Model file for the job. Use its own axes, mm. Give positions to 0.01 mm unless a question says otherwise; leave off trailing zeros. Answer as CSV lines item,"result". Start each with the question number.
Item 1: Pin check, flat tips, straight feed: pin 1 (0.8 mm diameter, centred on y = -234.5, z = 4, fed in from +X); pin 2 (0.8 mm diameter, centred on x = 4, y = -162, fed in from -Z); pin 3 (1.3 mm diameter, centred on x = -1.5, y = -277.5, fed in from +Z). Stop position of each tip, or through.
Item 2: Saw through at A-A on y = -317. State how many separate pieces and enclosed holes the cut face has, plus the area to 3 significant figures.
Item 3: Drill centre lines: L1, parallel to Z at x = 0, y = -327.5; L2, parallel to X at y = -107.5, z = 4.25; L3, parallel to Z at x = 3.25, y = -151. Where is each one in solid material? Low to high. Write a range as from..to.
from build123d import *

# Parameters (mm, degrees)
F0_R     = 2.1
F1_DEPTH = 460


with BuildPart() as f1:
    # F0 (on Front) → F1 (new body)
    with BuildSketch(Plane.XZ):
        with BuildLine():
            Line((-4.64, 10), (-9, 10))
            ThreePointArc((-9, 10), (-9.707107, 9.707107), (-10, 9))
            Line((-10, 9), (-10, 4.64))
            Line((-10, 4.64), (-8.2, 2.84))
            Line((-8.2, 2.84), (-8.2, 5.49934))
            Line((-8.2, 5.49934), (-6.56, 5.49934))
            Line((-6.56, 5.49934), (-3.90066, 2.84))
            Line((-3.90066, 2.84), (-3.90066, 0.15))
            Line((-3.90066, 0.15), (-3.75066, 0))
            Line((-3.75066, 0), (-3.90066, -0.15))
            Line((-3.90066, -0.15), (-3.90066, -2.84))
            Line((-3.90066, -2.84), (-6.56, -5.49934))
            Line((-6.56, -5.49934), (-8.2, -5.49934))
            Line((-8.2, -5.49934), (-8.2, -2.84))
            Line((-8.2, -2.84), (-10, -4.64))
            Line((-10, -4.64), (-10, -9))
            ThreePointArc((-10, -9), (-9.707107, -9.707107), (-9, -10))
            Line((-9, -10), (-4.64, -10))
            Line((-4.64, -10), (-2.84, -8.2))
            Line((-2.84, -8.2), (-5.49934, -8.2))
            Line((-5.49934, -8.2), (-5.49934, -6.56))
            Line((-5.49934, -6.56), (-2.84, -3.90066))
            Line((-2.84, -3.90066), (-0.15, -3.90066))
            Line((-0.15, -3.90066), (0, -3.75066))
            Line((0, -3.75066), (0.15, -3.90066))
            Line((0.15, -3.90066), (2.84, -3.90066))
            Line((2.84, -3.90066), (5.49934, -6.56))
            Line((5.49934, -6.56), (5.49934, -8.2))
            Line((5.49934, -8.2), (2.84, -8.2))
            Line((2.84, -8.2), (4.64, -10))
            Line((4.64, -10), (9, -10))
            ThreePointArc((9, -10), (9.707107, -9.707107), (10, -9))
            Line((10, -9), (10, -4.64))
            Line((10, -4.64), (8.2, -2.84))
            Line((8.2, -2.84), (8.2, -5.49934))
            Line((8.2, -5.49934), (6.56, -5.49934))
            Line((6.56, -5.49934), (3.90066, -2.84))
            Line((3.90066, -2.84), (3.90066, -0.15))
            Line((3.90066, -0.15), (3.75066, 0))
            Line((3.75066, 0), (3.90066, 0.15))
            Line((3.90066, 0.15), (3.90066, 2.84))
            Line((3.90066, 2.84), (6.56, 5.49934))
            Line((6.56, 5.49934), (8.2, 5.49934))
            Line((8.2, 5.49934), (8.2, 2.84))
            Line((8.2, 2.84), (10, 4.64))
            Line((10, 4.64), (10, 9))
            ThreePointArc((10, 9), (9.707107, 9.707107), (9, 10))
            Line((9, 10), (4.64, 10))
            Line((4.64, 10), (2.84, 8.2))
            Line((2.84, 8.2), (5.49934, 8.2))
            Line((5.49934, 8.2), (5.49934, 6.56))
            Line((5.49934, 6.56), (2.84, 3.90066))
            Line((2.84, 3.90066), (0.15, 3.90066))
            Line((0.15, 3.90066), (0, 3.75066))
            Line((0, 3.75066), (-0.15, 3.90066))
            Line((-0.15, 3.90066), (-2.84, 3.90066))
            Line((-2.84, 3.90066), (-5.49934, 6.56))
            Line((-5.49934, 6.56), (-5.49934, 8.2))
            Line((-5.49934, 8.2), (-2.84, 8.2))
            Line((-2.84, 8.2), (-4.64, 10))
        make_face()
        with BuildLine():
            Line((-8.2, -8.2), (-8.2, -6.71))
            ThreePointArc((-8.2, -6.71), (-8.156066, -6.603934), (-8.05, -6.56))
            Line((-8.05, -6.56), (-7.98749, -6.56))
            Line((-7.98749, -6.56), (-6.603934, -7.943556))
            ThreePointArc((-6.603934, -7.943556), (-6.571418, -7.992219), (-6.56, -8.049622))
            Line((-6.56, -8.049622), (-6.56, -8.05))
            ThreePointArc((-6.56, -8.05), (-6.603934, -8.156066), (-6.71, -8.2))
            Line((-6.71, -8.2), (-8.2, -8.2))
        make_face(mode=Mode.SUBTRACT)
        with BuildLine():
            ThreePointArc((6.71, -8.2), (6.603934, -8.156066), (6.56, -8.05))
            Line((6.56, -8.05), (6.56, -7.98749))
            Line((6.56, -7.98749), (7.943556, -6.603934))
            ThreePointArc((7.943556, -6.603934), (7.992219, -6.571418), (8.049622, -6.56))
            Line((8.049622, -6.56), (8.2, -6.56))
            Line((8.2, -6.56), (8.2, -8.05))
            ThreePointArc((8.2, -8.05), (8.156066, -8.156066), (8.05, -8.2))
            Line((8.05, -8.2), (6.71, -8.2))
        make_face(mode=Mode.SUBTRACT)
        with BuildLine():
            ThreePointArc((-8.2, 8.05), (-8.156066, 8.156066), (-8.05, 8.2))
            Line((-8.05, 8.2), (-6.71, 8.2))
            ThreePointArc((-6.71, 8.2), (-6.603934, 8.156066), (-6.56, 8.05))
            Line((-6.56, 8.05), (-6.56, 8.049622))
            ThreePointArc((-6.56, 8.049622), (-6.571418, 7.992219), (-6.603934, 7.943556))
            Line((-6.603934, 7.943556), (-7.943556, 6.603934))
            ThreePointArc((-7.943556, 6.603934), (-7.992219, 6.571418), (-8.049622, 6.56))
            Line((-8.049622, 6.56), (-8.05, 6.56))
            ThreePointArc((-8.05, 6.56), (-8.156066, 6.603934), (-8.2, 6.71))
            Line((-8.2, 6.71), (-8.2, 8.05))
        make_face(mode=Mode.SUBTRACT)
        Circle(F0_R, mode=Mode.SUBTRACT)
        with BuildLine():
            Line((8.2, 8.05), (8.2, 6.71))
            ThreePointArc((8.2, 6.71), (8.156066, 6.603934), (8.05, 6.56))
            Line((8.05, 6.56), (7.98749, 6.56))
            Line((7.98749, 6.56), (6.56, 7.98749))
            Line((6.56, 7.98749), (6.56, 8.05))
            ThreePointArc((6.56, 8.05), (6.603934, 8.156066), (6.71, 8.2))
            Line((6.71, 8.2), (8.05, 8.2))
            ThreePointArc((8.05, 8.2), (8.156066, 8.156066), (8.2, 8.05))
        make_face(mode=Mode.SUBTRACT)
    extrude(amount=F1_DEPTH)


solid = f1.part
Responses:
1,pin 1,"x = 9.76"
1,pin 2,"z = -9.76"
1,pin 3,"z = 3.9"
2,separate pieces,"1"
2,enclosed holes,"5"
2,area,"164 mm2"
3,L1,"-3.75..-2.1, 2.1..3.75"
3,L2,"-9.61..-8.2, -5.31..-3.19, 3.19..5.31, 8.2..9.61"
3,L3,"-8.61..-8.2, -4.31..4.31, 8.2..8.61"
